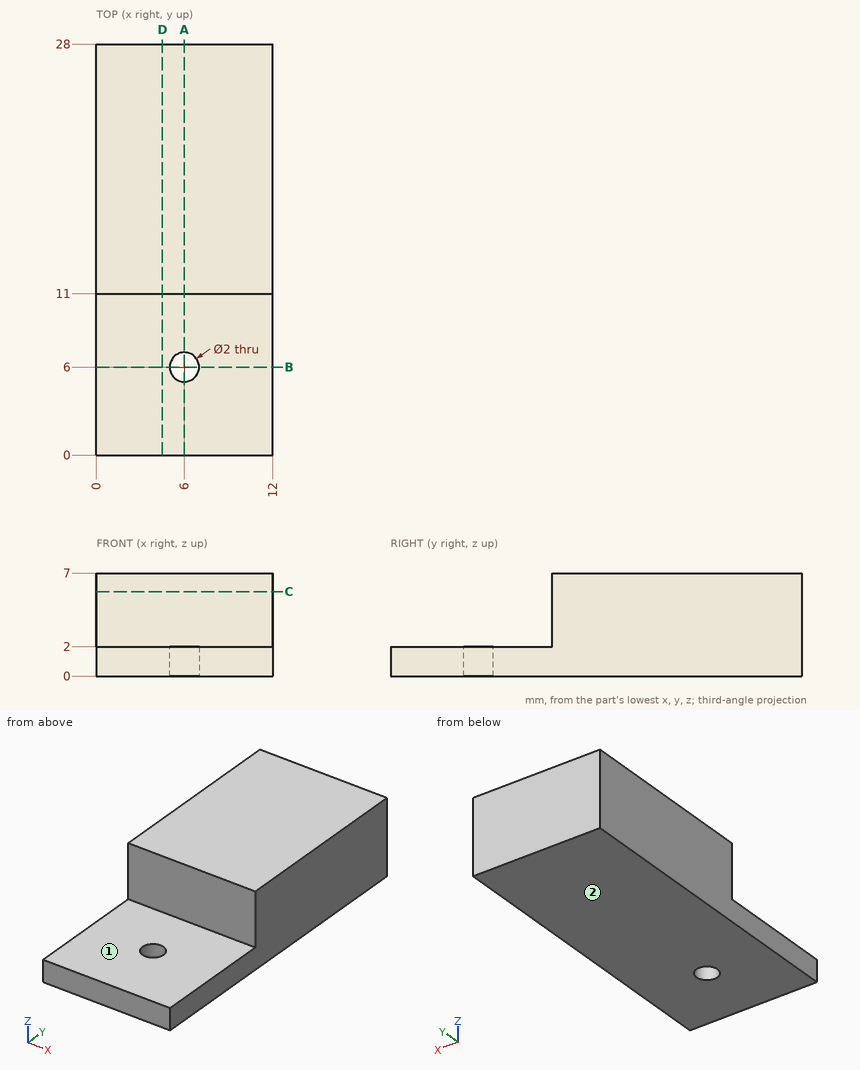
Geometry: see drawing. Coordinates: mm, zero at the bounding-box minimum. A direction names the side the tool comes from. Round coordinates to 2 decimals unless told otherwise and drop trailing zeros. Order: outer loops, then holes, each group sorted by start corner. A loop starts at its lowest first (then second) coordinate and runs counter-clockwise, first axis right, second up. Notation, with made-up numbers: (-8.5, -11.75) - (17.5, -11.75) arc R36 cw to (17.5, 25.25) - close; hole circle Ø3 at (64.5, -4.5). An arc over 180 degrees is marked (long way). Use a Markdown table: item, result. Add a question column.
1. Section query D-D (x = 4.5). Return the cut outline in (y, z), then the cut area to 3 significant figures.
2. Line query: probe 1 along Y at (x, z) = (6, 0.8); probe 2 along Z at (x, y) = (5.5, 1); probe 3 along Y at (x, z) = (8.25, 2.75). Output: solid intervals per line, ascending.
3. Section query A-A (x = 6). Return the cut outline in (y, z), then the cut area to 3 significant figures.
4. Section query B-B (y = 6). Return the cut outline in (x, z), then the cut area to 3 significant figures.
5. Section query C-C (z = 5.75). Return the cut outline in (x, y), then the cut area to 3 significant figures.
6. First-contact query: pin 1 (2 mm diameter, centred on x = 4.5, z = 6, fed in from -Y); pin 2 (1 mm diameter, centred on x = 9, y = 7, fed in from +Z). Flat tips, straight axial feed; report the tip coordinate or a pass-through.
7. Set-up query: the marked faces 1 and 2. Return all of +Z, -Z, +X, -X, +Y, -Y with unobstructed straight access to the full face (end or side cutting, diameter ignored); none if empty.
Derived:
| question | item | result |
|---|---|---|
| 1 | outline | (0, 0) - (28, 0) - (28, 7) - (11, 7) - (11, 2) - (0, 2) - close |
| 1 | area | 141 mm2 |
| 2 | probe 1 | 0 to 5, 7 to 28 |
| 2 | probe 2 | 0 to 2 |
| 2 | probe 3 | 11 to 28 |
| 3 | outline | (0, 0) - (5, 0) - (5, 2) - (0, 2) - close; (7, 0) - (28, 0) - (28, 7) - (11, 7) - (11, 2) - (7, 2) - close |
| 3 | area | 137 mm2 |
| 4 | outline | (0, 0) - (5, 0) - (5, 2) - (0, 2) - close; (7, 0) - (12, 0) - (12, 2) - (7, 2) - close |
| 4 | area | 20.0 mm2 |
| 5 | outline | (0, 11) - (12, 11) - (12, 28) - (0, 28) - close |
| 5 | area | 204 mm2 |
| 6 | pin 1 | y = 11 |
| 6 | pin 2 | z = 2 |
| 7 | face 1 | +Z, +X, -X, -Y |
| 7 | face 2 | -Z, +X, -X, +Y, -Y |
